from build123d import *

# Parameters (mm, degrees)
SKETCH1_W           = 30
SKETCH1_H           = 55
BOSS_EXTRUDE1_DEPTH = 20
CUT_EXTRUDE1_DEPTH  = 18
SKETCH3_W           = 2
SKETCH3_H           = 3
CUT_EXTRUDE2_DEPTH  = 21
SKETCH4_W           = 7
SKETCH4_H           = 16
CUT_EXTRUDE3_DEPTH  = 1
SKETCH5_R           = 1
CUT_EXTRUDE4_DEPTH  = 21
CUT_EXTRUDE5_DEPTH  = 1


with BuildPart() as part:
    # Sketch1 → Boss-Extrude1 (new body)
    with BuildSketch(Plane(origin=(0, 0, 0), x_dir=(1, 0, 0), z_dir=(0, 1, 0))):
        with Locations((15, 27.5)):
            Rectangle(SKETCH1_W, SKETCH1_H)
    extrude(amount=BOSS_EXTRUDE1_DEPTH)

    # Sketch2 → Cut-Extrude1 (cut)
    with BuildSketch(Plane(origin=(0, 20, 0), x_dir=(-1, 0, 0), z_dir=(0, 1, 0))):
        Polygon((-29, -52), (-1, -52), (-1, -49.101557188), (-2, -49.101557188), (-2, -2), (-28, -2), (-28, -49.101557188), (-29, -49.101557188), align=None)
    extrude(amount=-CUT_EXTRUDE1_DEPTH, mode=Mode.SUBTRACT)

    # Sketch3 → Cut-Extrude2 (cut, through all)
    with BuildSketch(Plane(origin=(0, 20, 0), x_dir=(-1, 0, 0), z_dir=(0, 1, 0))):
        with Locations((-4, -53.5)):
            Rectangle(SKETCH3_W, SKETCH3_H)
        with Locations((-26, -53.5)):
            Rectangle(SKETCH3_W, SKETCH3_H)
    extrude(amount=-CUT_EXTRUDE2_DEPTH, mode=Mode.SUBTRACT)

    # Sketch4 → Cut-Extrude3 (cut)
    with BuildSketch(Plane(origin=(0, 0, -55), x_dir=(-1, 0, 0), z_dir=(0, 0, -1))):
        with Locations((-19.5, 10)):
            Rectangle(SKETCH4_W, SKETCH4_H)
        with Locations((-10.5, 10)):
            Rectangle(SKETCH4_W, SKETCH4_H)
    extrude(amount=-CUT_EXTRUDE3_DEPTH, mode=Mode.SUBTRACT)

    # Sketch5 → Cut-Extrude4 (cut, through all)
    with BuildSketch(Plane.XZ):
        with Locations((6.5, -14)):
            Circle(SKETCH5_R)
        with Locations((23.5, -14)):
            Circle(SKETCH5_R)
        with Locations((6.5, -35)):
            Circle(SKETCH5_R)
        with Locations((23.5, -35)):
            Circle(SKETCH5_R)
    extrude(amount=-CUT_EXTRUDE4_DEPTH, mode=Mode.SUBTRACT)

    # Sketch6 → Cut-Extrude5 (cut)
    with BuildSketch(Plane.XZ):
        Polygon((4.871763373, 0), (4.871763373, -2.932893163), (7.8857023, -2.932893163), (7.8857023, -12.114893151), (12.091198477, -12.114893151), (12.091198477, -13.867183225), (17.908801523, -13.867183225), (17.908801523, -12.114893151), (22.1142977, -12.114893151), (22.1142977, -2.932893163), (25.128236627, -2.932893163), (25.128236627, 0), align=None)
        Polygon((0, -20.87634352), (3.680206122, -20.87634352), (3.680206122, -22.698725197), (6.834328255, -22.698725197), (6.834328255, -20.87634352), (23.165671745, -20.87634352), (23.165671745, -22.698725197), (26.319793878, -22.698725197), (26.319793878, -20.87634352), (30, -20.87634352), (30, -28.376145037), (26.319793878, -28.376145037), (26.319793878, -26.203305345), (23.165671745, -26.203305345), (23.165671745, -28.376145037), (6.834328255, -28.376145037), (6.834328255, -26.203305345), (3.680206122, -26.203305345), (3.680206122, -28.376145037), (0, -28.376145037), align=None)
        Polygon((0, -39.310435098), (3.680206122, -44.006572497), (5.712862608, -44.006572497), (6.834328255, -42.885106849), (6.834328255, -39.801076319), (23.165671745, -39.801076319), (23.165671745, -42.885106849), (24.287137392, -44.006572497), (26.319793878, -44.006572497), (30, -39.310435098), (30, -55), (28.159896939, -55), (28.159896939, -51.43628241), (1.840103061, -51.43628241), (1.840103061, -55), (0, -55), align=None)
    extrude(amount=-CUT_EXTRUDE5_DEPTH, mode=Mode.SUBTRACT)


solid = part.part
The model under review builds one solid part; all positions refer to its coordinate system, in mm. A direction names the side the tool comes from. Give positions to 0.01 mm unless a question says otherwise; leave off trailing zeros. Loops run counter-clockwise (first coordinate to the right, second up) from the corner with the lowest first, then second, coordinate; pieces in that order, holes last. Notation, with made-up numbers: (-7, -10) -> (4, -10) arc R29 ccw to (4, 19) -> close; hole circle Ø9 at (67, -8.75). An arc over 180 degrees is marked (long way). Put each result on its own line as item: value. Start each with the question number.
1. We need section A-A on z = -35. State the section outline as (x, y) points, then the cut area to 3 significant figures.
2. We need section D-D on z = -16. State the section outline as (x, y) points.
3. Wall thickness on probe 1 along Z at (x, y) = (6.5, 1.3); probe 2 along X at (y, z) = (15.75, -44); probe 3 along Z at (x, y) = (22.5, 13): over which ranges is each line inside the solid? List them lowest first.
4. We need section C-C on z = -8. State the section outline as (x, y) points.
5. Clearance check with flat-ended pins moving along their axes: P1, Ø0.5, axis at x = 28.5, y = 0.5, coming from the -Z side; P2, Ø1.2, axis at x = 23.5, z = -35, coming from the -Y side; P3, Ø2.5, axis at x = 23.5, z = -14, coming from the +Y side; P4, Ø5.5, axis at x = 11, y = 7.5, coming from the -Z side. State where each tip first meets the part, or that it passes through.
6. For faces 4 (the face through (1.814, 0.493, -41.626)), 5 (the face through (25.3, 0.5, -44.007)), 6 (the face through (6.834, 0.5, -27.3)), 7 (the face through (19.5, 18, -54.5)), 8 (the face through (5, 10, -54)), list the 3-axis set-ups (+Z, -Z, +X, -X, +Y, -Y) from which the entire face can be reached by the end or side of a thin tool; tool diameter is ignored.
7. We need section B-B on y = 6.75. State the section outline as (x, z) points, then the cut area to 3 significant figures.
8. Mouldability with a two-part tool opening along Z and no side actions: class faces 1 (the face through (2, 11, -26)), 2 (the face through (23.6, 0.5, -2.933)), 3 (the face through (4.872, 0.5, -1.4)) as released by +Z, released by -Z, zero draft, split by the parting line, or undercut.
Determined:
1. outline: (0, 0) -> (5.5, 0) -> (5.5, 2) -> (2, 2) -> (2, 20) -> (0, 20) -> close; (7.5, 0) -> (22.5, 0) -> (22.5, 2) -> (7.5, 2) -> close; (24.5, 0) -> (30, 0) -> (30, 20) -> (28, 20) -> (28, 2) -> (24.5, 2) -> close
1. area: 124 mm^2
2. outline: (0, 0) -> (30, 0) -> (30, 20) -> (28, 20) -> (28, 2) -> (2, 2) -> (2, 20) -> (0, 20) -> close
3. probe 1: -55 to -36, -34 to -15, -13 to 0
3. probe 2: 0 to 2, 28 to 30
3. probe 3: -54 to -52, -2 to 0
4. outline: (0, 0) -> (7.89, 0) -> (7.89, 1) -> (22.11, 1) -> (22.11, 0) -> (30, 0) -> (30, 20) -> (28, 20) -> (28, 2) -> (2, 2) -> (2, 20) -> (0, 20) -> close
5. P1: z = -41.54
5. P2: through
5. P3: y = 2
5. P4: z = -54
6. face 4: -X, -Y
6. face 5: +X, -X, -Y
6. face 6: -Y
6. face 7: -Z
6. face 8: -Z, +Y, -Y
7. outline: (0, -55) -> (3, -55) -> (3, -52) -> (1, -52) -> (1, -49.1) -> (2, -49.1) -> (2, -2) -> (28, -2) -> (28, -49.1) -> (29, -49.1) -> (29, -52) -> (27, -52) -> (27, -55) -> (30, -55) -> (30, 0) -> (0, 0) -> close; (5, -55) -> (7, -55) -> (7, -54) -> (14, -54) -> (14, -55) -> (16, -55) -> (16, -54) -> (23, -54) -> (23, -55) -> (25, -55) -> (25, -52) -> (5, -52) -> close
7. area: 318 mm^2
8. face 1: undercut
8. face 2: released by +Z
8. face 3: zero draft
